Check sheet for the modelled part. Datum: model origin and axes. Units: mm. Face numbers are marked on the shaded views. Give positions to 0.01 mm unless a question says otherwise; leave off trailing zeros. Write each loop counter-clockwise with the first axis right and the second up, starting at its lowest first coordinate (ties: lowest second). Pieces come first, ordered by that corner, then holes. Notation, with made-up numbers: (-8.5, 87) -> (-3.5, 87) arc R14 ccw to (-3.5, 97) -> close; hole circle Ø6 at (85.5, 43). An arc over 180 degrees is marked (long way). Answer as a JSON object with one key per item and string values.
from build123d import *

# Parameters (mm, degrees)
SKETCH1_R           = 0.95
BOSS_EXTRUDE1_DEPTH = 2.625
SKETCH2_W           = 37.893298516
SKETCH2_H           = 2.75
CUT_EXTRUDE1_DEPTH  = 13.625
BOSS_EXTRUDE2_DEPTH = 5.25


with BuildPart() as part:
    # Sketch1 → Boss-Extrude1 (new, symmetric)
    with BuildSketch(Plane.XY):
        with BuildLine():
            Line((17, 2), (0.197906371, 3.334283906))
            ThreePointArc((0.197906371, 3.334283906), (0, 3.342129603), (-0.197906371, 3.334283906))
            Line((-0.197906371, 3.334283906), (-17, 2))
            ThreePointArc((-17, 2), (-19, 0), (-17, -2))
            Line((-17, -2), (-0.389436602, -4.619481551))
            ThreePointArc((-0.389436602, -4.619481551), (0, -4.65), (0.389436602, -4.619481551))
            Line((0.389436602, -4.619481551), (17, -2))
            ThreePointArc((17, -2), (19, 0), (17, 2))
        make_face()
        with Locations(Location((-17, 0, 0), (0, 0, 180))):
            Circle(SKETCH1_R, mode=Mode.SUBTRACT)
        with Locations(Location((17, 0, 0), (0, 0, 180))):
            Circle(SKETCH1_R, mode=Mode.SUBTRACT)
        with Locations(Location((0, -1.75, 0), (0, 0, 180))):
            Circle(SKETCH1_R, mode=Mode.SUBTRACT)
    extrude(amount=BOSS_EXTRUDE1_DEPTH, both=True)

    # Sketch2 → Cut-Extrude1 (cut, symmetric)
    with BuildSketch(Plane(origin=(0.264362283, 3.329006525, 0), x_dir=(0.996861721065102, -0.07916254843752263, 0), z_dir=(0.07916254843752263, 0.996861721065102, 0))):
        Rectangle(SKETCH2_W, SKETCH2_H)
    extrude(amount=CUT_EXTRUDE1_DEPTH, both=True, mode=Mode.SUBTRACT)


with BuildPart() as cut_extrude1_piece_1:
    # of the separate pieces the step leaves, piece 1, a body of its own (cut_extrude1_pieces)
    add(part.part.solids().sort_by_distance((17, 2, 2.625))[0])



with BuildPart() as cut_extrude1_piece_2:
    # of the separate pieces the step leaves, piece 2, a body of its own (cut_extrude1_pieces)
    add(part.part.solids().sort_by_distance((17, 2, -1.375))[0])


with BuildPart() as cut_extrude1_piece_1_1:
    add(cut_extrude1_piece_1.part)

    add(cut_extrude1_piece_2.part)  # Boss-Extrude2 merges Cut-Extrude1 piece 2
    # Sketch3 → Boss-Extrude2 (add)
    with BuildSketch(Plane.XY.offset(2.625)):
        with BuildLine():
            Line((6.692125271, -1.355773858), (11.670347401, 1.620348522))
            ThreePointArc((11.670347401, 1.620348522), (12.493210627, 1.413234754), (12.286096859, 0.590371529))
            Line((12.286096859, 0.590371529), (7.307874729, -2.385750851))
            ThreePointArc((7.307874729, -2.385750851), (6.485011504, -2.178637083), (6.692125271, -1.355773858))
        make_face()
    extrude(amount=-BOSS_EXTRUDE2_DEPTH)


solid = cut_extrude1_piece_1_1.part
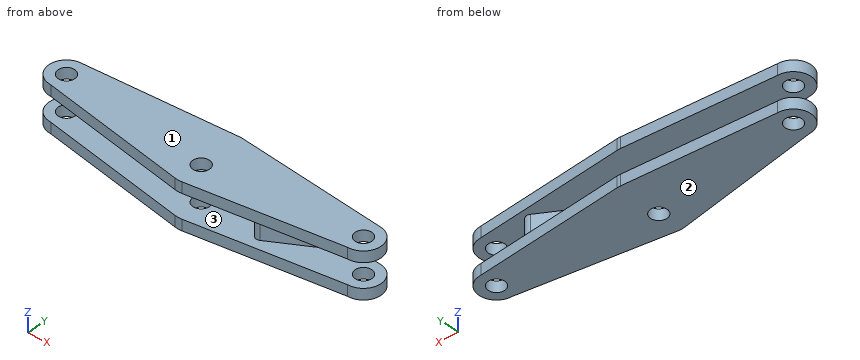
1. Sectioned sample at D-D, the plane z = 0.75. Enter the section's corners in (x, y).
Determined:
{"outline": "(6.69, -1.36) arc R0.6 ccw to (7.31, -2.39) -> (12.29, 0.59) arc R0.6 ccw to (11.67, 1.62) -> close"}
2. Sectioned sample at A-A, the plane y = -4. Enter the section's corners in (x, z) (3 decimals), plus the area to 3 significant figures.
Determined:
{"outline": "(-4.318, -2.625) -> (4.318, -2.625) -> (4.318, -1.375) -> (-4.318, -1.375) -> close; (-4.318, 1.375) -> (4.318, 1.375) -> (4.318, 2.625) -> (-4.318, 2.625) -> close", "area": "21.6 mm^2"}
3. Sectioned sample at C-C, the plane z = -2.1. Enter the section's corners in (x, y).
Determined:
{"outline": "(-17, -2) -> (-0.39, -4.62) arc R2.5 ccw to (0.39, -4.62) -> (17, -2) arc R2 ccw to (17, 2) -> (0.2, 3.33) arc R2.5 ccw to (-0.2, 3.33) -> (-17, 2) arc R2 ccw to start; hole circle Ø1.9 at (-17, 0); hole circle Ø1.9 at (0, -1.75); hole circle Ø1.9 at (17, 0)"}
4. Sectioned sample at B-B, the plane x = -5.5. Enter the section's corners in (y, z) (3 decimals).
Determined:
{"outline": "(-3.814, -2.625) -> (2.913, -2.625) -> (2.913, -1.375) -> (-3.814, -1.375) -> close; (-3.814, 1.375) -> (2.913, 1.375) -> (2.913, 2.625) -> (-3.814, 2.625) -> close"}
5. Mould release check, pull along Z, two halves, no side actions. Record for the marked faces 1, 2 and 3: released by +Z, released by -Z, zero draft, split by the parting line, or undercut.
Determined:
{"face 1": "released by +Z", "face 2": "released by -Z", "face 3": "undercut"}
6. Scan lines: L1, parallel to Z at x = -1, y = -3.5 (3 decimals); L2, parallel to Y at x = 0, z = 2.2; L3, parallel to Y at x = -17, z = 2.2. Record each from-to range of solid material in increasing order. Write a range as [from, to].
Determined:
{"L1": "[-2.625, -1.375], [1.375, 2.625]", "L2": "[-4.65, -2.7], [-0.8, 3.34]", "L3": "[-2, -0.95], [0.95, 2]"}
7. Go/stop test with flat-tipped pins: P1, Ø2, axis at x = 17, y = 0, coming from the +Z side (3 decimals); P2, Ø1.5, axis at x = -10.5, z = -1, coming from the +Y side. Record where each tip stops, or that it passes through.
Determined:
{"P1": "z = 2.625", "P2": "y = 2.57"}
